Geometry check sheet. Reference: the model listing, model coordinates, mm. A direction names the side the tool comes from. Give positions to 0.01 mm unless a question says otherwise; leave off trailing zeros. Loops run counter-clockwise (first coordinate to the right, second up) from the corner with the lowest first, then second, coordinate; pieces in that order, holes last.
```python
from build123d import *

# Parameters (mm, degrees)
SKETCH1_R           = 39
BOSS_EXTRUDE1_DEPTH = 6.35
SKETCH2_R           = 15
CUT_EXTRUDE1_DEPTH  = 6.35
SKETCH3_R           = 20
SKETCH3_R_2         = 15
BOSS_EXTRUDE2_DEPTH = 8.65
SKETCH4_R           = 20
SKETCH4_R_2         = 15
BOSS_EXTRUDE3_DEPTH = 45
SKETCH5_R           = 3.25
CUT_EXTRUDE2_DEPTH  = 45


with BuildPart() as part:
    # Sketch1 → Boss-Extrude1 (new body)
    with BuildSketch(Plane(origin=(0, 0, 0), x_dir=(0, 0, -1), z_dir=(1, 0, 0))):
        Circle(SKETCH1_R)
    extrude(amount=BOSS_EXTRUDE1_DEPTH)

    # Sketch2 → Cut-Extrude1 (cut)
    with BuildSketch(Plane(origin=(6.35, 0, 0), x_dir=(0, 0, -1), z_dir=(1, 0, 0))):
        Circle(SKETCH2_R)
    extrude(amount=-CUT_EXTRUDE1_DEPTH, mode=Mode.SUBTRACT)

    # Sketch3 → Boss-Extrude2 (add)
    with BuildSketch(Plane(origin=(6.35, 0, 0), x_dir=(0, 0, -1), z_dir=(1, 0, 0))):
        Circle(SKETCH3_R)
        Circle(SKETCH3_R_2, mode=Mode.SUBTRACT)
    extrude(amount=BOSS_EXTRUDE2_DEPTH)

    # Sketch4 → Boss-Extrude3 (add)
    with BuildSketch(Plane.ZY):
        Circle(SKETCH4_R)
        Circle(SKETCH4_R_2, mode=Mode.SUBTRACT)
    extrude(amount=BOSS_EXTRUDE3_DEPTH)

    # Sketch5 → Cut-Extrude2 (cut)
    with BuildSketch(Plane.ZY):
        with Locations((0, 30.27)):
            Circle(SKETCH5_R)
        with Locations((-30.27, 0)):
            Circle(SKETCH5_R)
        with Locations((30.27, 0)):
            Circle(SKETCH5_R)
        with Locations((0, -30.27)):
            Circle(SKETCH5_R)
    extrude(amount=-CUT_EXTRUDE2_DEPTH, mode=Mode.SUBTRACT)


solid = part.part
```
1) Depth check by flat-ended pin: P1, Ø2, axis at x = -21, y = -19, coming from the -Z side; P2, Ø5, axis at y = 0, z = -30.27, coming from the +X side; P3, Ø2, axis at x = -30, y = -1, coming from the +Z side; P4, Ø6, axis at y = -20, z = -30, coming from the +X side. Enter the tip coordinate at first touch or a pass-through.
2) Sectioned sample at D-D on y = 13. Enter the section's corners in (x, z), plus the area to 3 significant figures.
3) Scan lines: line 1 along Y through (x, z) = (4, 0); line 2 along Y through (x, z) = (-10, 0); line 3 along X through (y, z) = (26, 4). Record each from-to range of solid material in increasing order.
4) Sectioned sample at C-C on x = -29. Enter the section's corners in (y, z).
5) Tool access check on faces 1 (the flat face through (0, -17, -17)), 2 (the cylindrical face through (10.614, -19.524, 4.336)), 3 (the cylindrical face through (3.131, 38.668, 5.077)). Record the directions out of +Z, -Z, +X, -X, +Y, -Y that give a thin tool (end or side, any length) a straight path to the whole face; none if there is none.
6) Sectioned sample at A-A on z = 0. Enter the section's corners in (x, y).
7) Mould release check, pull along Y, two halves, no side actions. Record for faces 4 (the cylindrical face through (3.131, -33.443, -0.705)), 5 (the cylindrical face through (-22.185, -19.524, -4.336)), 6 (the flat face through (-45, 15, 3)): +Y half, -Y half, draft (parallel to the pull), parting line (faces both ways), or undercut.
Determined:
1. P1: stops at z = -8.72
1. P2: passes through
1. P3: stops at z = 20
1. P4: stops at x = 6.35
2. outline: (-45, -15.2) - (0, -15.2) - (0, -36.77) - (6.35, -36.77) - (6.35, -15.2) - (15, -15.2) - (15, -7.48) - (-45, -7.48) - close; (-45, 7.48) - (15, 7.48) - (15, 15.2) - (6.35, 15.2) - (6.35, 36.77) - (0, 36.77) - (0, 15.2) - (-45, 15.2) - close
2. area: 1,200 mm2
3. line 1: y = -39 to -33.52, -27.02 to -15, 15 to 27.02, 33.52 to 39
3. line 2: y = -20 to -15, 15 to 20
3. line 3: x = 0 to 6.35
4. outline: circle Ø40 at (0, 0); hole circle Ø30 at (0, 0)
5. face 1: -X
5. face 2: +X
5. face 3: +X, -X
6. outline: (-45, -20) - (0, -20) - (0, -27.02) - (6.35, -27.02) - (6.35, -20) - (15, -20) - (15, -15) - (-45, -15) - close; (-45, 15) - (15, 15) - (15, 20) - (6.35, 20) - (6.35, 27.02) - (0, 27.02) - (0, 20) - (-45, 20) - close; (0, -39) - (6.35, -39) - (6.35, -33.52) - (0, -33.52) - close; (0, 33.52) - (6.35, 33.52) - (6.35, 39) - (0, 39) - close
7. face 4: undercut
7. face 5: parting line
7. face 6: draft
